Source: CAD feature listing. Evaluate the final solid. Frame: model axes, mm. A direction names the side the tool comes from. Round coordinates to 2 decimals unless told otherwise and drop trailing zeros. Loops run counter-clockwise (first coordinate to the right, second up) from the corner with the lowest first, then second, coordinate; pieces in that order, holes last. Notation, with made-up numbers: (66.25, 46) - (90.25, 46) arc R28 cw to (90.25, 82) - close; hole circle Ø4 at (33, 20). An arc over 180 degrees is marked (long way). Write item = value, one per line. Start each with the question number.
from build123d import *

# Parameters (mm, degrees)
SKETCH_1_W          = 40
SKETCH_1_H          = 28
SKETCH_1_R          = 2
EXTRUDE_1_DEPTH     = 51.5
SKETCH_2_W          = 22.5
SKETCH_2_H          = 20
EXTRUDE_2_DEPTH     = 18
SKETCH_3_W          = 13.5
SKETCH_3_H          = 7
CUT_EXTRUDE_1_DEPTH = 12
SKETCH_4_W          = 22.5
SKETCH_4_H          = 1
CUT_EXTRUDE_2_DEPTH = 12
SKETCH_5_W          = 7
SKETCH_5_H          = 12
CUT_EXTRUDE_3_DEPTH = 7


with BuildPart() as part:
    # 草图1 → 凸台-拉伸1 (new body)
    with BuildSketch(Plane.XY):
        Rectangle(SKETCH_1_W, SKETCH_1_H)
        with Locations((-17, 11)):
            Circle(SKETCH_1_R, mode=Mode.SUBTRACT)
        with Locations((17, 11)):
            Circle(SKETCH_1_R, mode=Mode.SUBTRACT)
        with Locations((-17, -11)):
            Circle(SKETCH_1_R, mode=Mode.SUBTRACT)
        with Locations((17, -11)):
            Circle(SKETCH_1_R, mode=Mode.SUBTRACT)
    extrude(amount=EXTRUDE_1_DEPTH)

    # 草图2 → 凸台-拉伸2 (add)
    with BuildSketch(Plane.XY.offset(51.5)):
        with Locations((0, 4)):
            Rectangle(SKETCH_2_W, SKETCH_2_H)
    extrude(amount=EXTRUDE_2_DEPTH)

    # 草图3 → 切除-拉伸1 (cut)
    with BuildSketch(Plane.XZ.offset(6)):
        with Locations((0, 55)):
            Rectangle(SKETCH_3_W, SKETCH_3_H)
    extrude(amount=-CUT_EXTRUDE_1_DEPTH, mode=Mode.SUBTRACT)

    # 草图4 → 切除-拉伸2 (cut)
    with BuildSketch(Plane.XZ.offset(6)):
        with Locations((0, 62)):
            Rectangle(SKETCH_4_W, SKETCH_4_H)
    extrude(amount=-CUT_EXTRUDE_2_DEPTH, mode=Mode.SUBTRACT)

    # 草图5 → 切除-拉伸3 (cut)
    with BuildSketch(Plane.XY.offset(69.5)):
        Rectangle(SKETCH_5_W, SKETCH_5_H)
    extrude(amount=-CUT_EXTRUDE_3_DEPTH, mode=Mode.SUBTRACT)


solid = part.part
(1) Cut plane D-D (y = 11). Output: boundary loops of the cut face in (x, z).
(2) Mould query, pull axis Z, two halves, no side actions, for faces 1 (the face through (-7, -6, 66)), 2 (the face through (6.75, 0, 55)), 3 (the face through (0, 0, 0)). Classes: +Z half, -Z half, draft (parallel to the pull), parting line (faces both ways), or undercut.
(3) Access query for faces 4 (the face through (3.5, 0, 66)), 5 (the face through (-6.75, 0, 55)), 6 (the face through (-7, 0, 62.5)). Directions: +Z, -Z, +X, -X, +Y, -Y. A direction counts if a zero-diameter tool reaches every point of the face in a straight line with its end or side. Return the directions, or none.
(4) Cut plane C-C (z = 18.5). Output: boundary loops of the cut face in (x, y), and give its area (3 significant figures).
(5) Pin query (flat end, axial travel): P1, Ø5.5, axis at x = -7.5, z = 66, coming from the -Y side; P2, Ø3.5, axis at y = -2, z = 53.5, coming from the -X side; P3, Ø5, axis at x = 4.5, y = 0, coming from the -Z side; P4, Ø4.5, axis at x = 17, y = 11, coming from the +Z side. Return the tip coordinate at first contact, or that it passes through.
(6) Cut plane A-A (y = -3.5). Output: boundary loops of the cut face in (x, z), and give its area (3 significant figures).
(7) Cut plane B-B (x = -17). Output: boundary loops of the cut face in (y, z).
(8) Material intervals for line 1 along Y through (x, z) = (-17, 17.5); line 2 along Z through (x, y) = (-10, 4.5); line 3 along X through (y, z) = (-12, 24.5), sorted ascending. Write a range as from..to.
Solution:
q1.outline = (-20, 0) - (-19, 0) - (-19, 51.5) - (-20, 51.5) - close; (-15, 0) - (15, 0) - (15, 51.5) - (11.25, 51.5) - (11.25, 69.5) - (-11.25, 69.5) - (-11.25, 51.5) - (-15, 51.5) - close; (19, 0) - (20, 0) - (20, 51.5) - (19, 51.5) - close
q2.face_1 = draft
q2.face_2 = undercut
q2.face_3 = -Z half
q3.face_4 = +Z, -Y
q3.face_5 = -Y
q3.face_6 = +X, -X, -Y
q4.outline = (-20, -14) - (20, -14) - (20, 14) - (-20, 14) - close; hole circle Ø4 at (-17, -11); hole circle Ø4 at (-17, 11); hole circle Ø4 at (17, -11); hole circle Ø4 at (17, 11)
q4.area = 1,070 mm^2
q5.P1 = -6
q5.P2 = -11.25
q5.P3 = 0
q5.P4 = 51.5
q6.outline = (-20, 0) - (20, 0) - (20, 51.5) - (11.25, 51.5) - (11.25, 61.5) - (-11.25, 61.5) - (-11.25, 51.5) - (-20, 51.5) - close; (-11.25, 62.5) - (-3.5, 62.5) - (-3.5, 69.5) - (-11.25, 69.5) - close; (3.5, 62.5) - (11.25, 62.5) - (11.25, 69.5) - (3.5, 69.5) - close; hole (-6.75, 51.5) - (6.75, 51.5) - (6.75, 58.5) - (-6.75, 58.5) - close
q6.area = 2,300 mm^2
q7.outline = (-14, 0) - (-13, 0) - (-13, 51.5) - (-14, 51.5) - close; (-9, 0) - (9, 0) - (9, 51.5) - (-9, 51.5) - close; (13, 0) - (14, 0) - (14, 51.5) - (13, 51.5) - close
q8.line_1 = -14..-13, -9..9, 13..14
q8.line_2 = 0..61.5, 62.5..69.5
q8.line_3 = -20..-18.73, -15.27..15.27, 18.73..20
